The model under review builds one solid part; all positions refer to its coordinate system, in mm. Face numbers are marked on the shaded views. Coordinates: 2 decimals unless noted, no trailing zeros. Write each loop counter-clockwise with the first axis right and the second up, starting at its lowest first coordinate (ties: lowest second). Pieces come first, ordered by that corner, then holes. Notation, with made-up numbers: (-15.5, 75.25) - (38.5, 75.25) arc R7 cw to (38.5, 87.25) - close; hole circle Ø6 at (81.25, -38). An arc over 180 degrees is marked (long way). Put each result on its own line as item: value. Start each with the question number.
Item 1: Consider section C-C on y = -57.5. Give the boundary of the cut face in (x, z).
Item 2: Consider section B-B on x = 0. Give the boundary of the cut face in (y, z).
Item 3: Consider section D-D on x = 11. Give the boundary of the cut face in (y, z), then the cut area to 3 significant figures.
Item 4: For pin 1 (1 mm diameter, centred on x = -9.5, y = -26, fed in from +Z); pin 2 (2 mm diameter, centred on x = 0, z = -6.5, fed in from -Y); pin 3 (5 mm diameter, centred on x = -8, y = -27.5, fed in from +Z); pin 4 (4 mm diameter, centred on y = -29.5, z = -6.5, fed in from -X), all flat-tipped, find the tip position at first contact; note any pin that passes through.
Item 5: Consider section A-A on z = 0. Give the boundary of the cut face in (x, y).
Item 6: To check wall thickness, follow L1, parallel to Z at x = 0, y = -11; L2, parallel to Y at x = -3.25, z = -9.25; L3, parallel to Z at x = 0, y = -49.5. State the ranges of each line that lie inside material, in increasing order. Write a range as [from, to].
Item 7: Mouldability with a two-part tool opening along X and no side actions: class the marked faces 1, 2 and 3 as pulls with the +X half, pulls with the -X half, needs draft (parallel to the pull), parting line crosses it, or undercut.
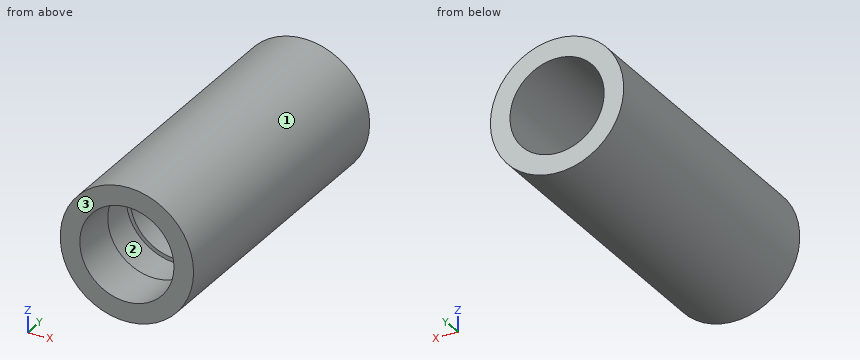
```python
from build123d import *

# Parameters (mm, degrees)
F0_R     = 13.45
F0_R_2   = 9.5
F1_DEPTH = 63
F2_W     = 8
F2_H     = 0.8


with BuildPart() as f1:
    # F0 (on Front) → F1 (new body)
    with BuildSketch(Plane.XZ):
        Circle(F0_R)
        Circle(F0_R_2, mode=Mode.SUBTRACT)
    extrude(amount=F1_DEPTH)

    # F2 (on Right) → F3 (revolve, cut)
    with BuildSketch(Plane.YZ):
        with Locations((-49, 9.9)):
            Rectangle(F2_W, F2_H)
    revolve(axis=Axis((0, -31.5, 0), (0, -1, 0)), mode=Mode.SUBTRACT)


solid = f1.part
```
Report:
1. outline: circle Ø26.9 at (0, 0); hole circle Ø19 at (0, 0)
2. outline: (-63, -13.45) - (0, -13.45) - (0, -9.5) - (-45, -9.5) - (-45, -10.3) - (-53, -10.3) - (-53, -9.5) - (-63, -9.5) - close; (-63, 9.5) - (-53, 9.5) - (-53, 10.3) - (-45, 10.3) - (-45, 9.5) - (0, 9.5) - (0, 13.45) - (-63, 13.45) - close
3. outline: (-63, -7.74) - (0, -7.74) - (0, 7.74) - (-63, 7.74) - close
3. area: 975 mm²
4. pin 1: z = 10
4. pin 2: through
4. pin 3: z = 12.27
4. pin 4: x = -12.67
5. outline: (-13.45, -63) - (-9.5, -63) - (-9.5, -53) - (-10.3, -53) - (-10.3, -45) - (-9.5, -45) - (-9.5, 0) - (-13.45, 0) - close; (9.5, -63) - (13.45, -63) - (13.45, 0) - (9.5, 0) - (9.5, -45) - (10.3, -45) - (10.3, -53) - (9.5, -53) - close
6. L1: [-13.45, -9.5], [9.5, 13.45]
6. L2: [-63, -53], [-45, 0]
6. L3: [-13.45, -10.3], [10.3, 13.45]
7. face 1: parting line crosses it
7. face 2: undercut
7. face 3: needs draft
